Can you work these out from the model? Positions are in its coordinate system, mm. Face numbers are marked on the shaded views. A direction names the side the tool comes from. Give positions to 0.01 mm unless a question says otherwise; leave off trailing zeros. Order: outer loops, then holes, each group sorted by start corner. A loop starts at its lowest first (then second) coordinate and runs counter-clockwise, first axis right, second up. Notation, with made-up numbers: (23, 53) - (69, 53) arc R27 cw to (69, 75) - close; hole circle Ø3 at (81, -6.75). An arc over 180 degrees is marked (long way). Write each question's results on one line, items separated by ' | '. Start each with the question number.
from build123d import *

# Parameters (mm, degrees)
SKETCH1_W                    = 838.2
SKETCH1_H                    = 101.6
BASE_FLANGE1_DEPTH           = 3.175
EDGE_FLANGE1_STRIP_W         = 19.05
EDGE_FLANGE1_STRIP_H         = 3.175
EDGE_FLANGE1_STRIP_CUT_DEPTH = 838.2
EDGE_FLANGE1_DEPTH           = 838.2


# Sheet-metal steps are written as plain solids
with BuildPart() as part:
    # Sketch1 → Base-Flange1 (new body)
    with BuildSketch(Plane(origin=(0, 0, 0), x_dir=(1, 0, 0), z_dir=(0, 1, 0))):
        with Locations((419.1, 50.8)):
            Rectangle(SKETCH1_W, SKETCH1_H)
    extrude(amount=-BASE_FLANGE1_DEPTH)

    # Edge-Flange1 strip (across the edge) → Edge-Flange1 strip cut (cut)
    with BuildSketch(Plane(origin=(0, 0, 0), x_dir=(0, 0, -1), z_dir=(1, 0, 0))):
        with Locations((-3.175, -1.5875)):
            Rectangle(EDGE_FLANGE1_STRIP_W, EDGE_FLANGE1_STRIP_H)
    extrude(amount=EDGE_FLANGE1_STRIP_CUT_DEPTH, mode=Mode.SUBTRACT)

    # Edge-Flange1 section (across the edge) → Edge-Flange1 (add)
    with BuildSketch(Plane(origin=(0, 0, 0), x_dir=(0, 0, -1), z_dir=(1, 0, 0))):
        with BuildLine():
            Line((0, 3.175), (0, 38.1))
            Line((0, 38.1), (3.175, 38.1))
            Line((3.175, 38.1), (3.175, 3.175))
            ThreePointArc((3.175, 3.175), (4.10493597, 0.92993597), (6.35, 0))
            Line((6.35, 0), (6.35, -3.175))
            ThreePointArc((6.35, -3.175), (1.859871939, -1.315128061), (0, 3.175))
        make_face()
    extrude(amount=EDGE_FLANGE1_DEPTH)


solid = part.part
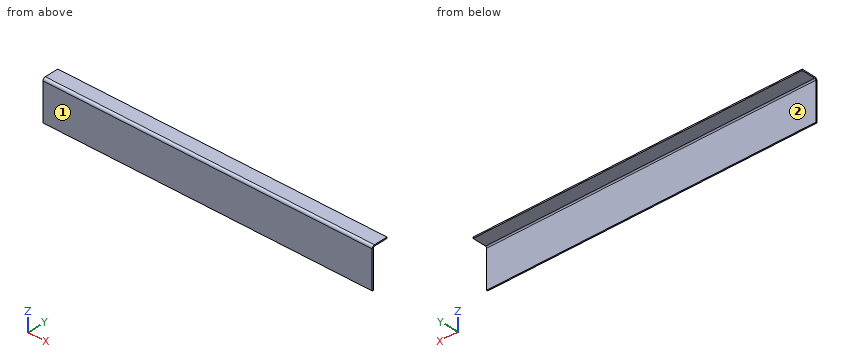
Q1. Will these pins go through, and if not, where does the flat tip stop? P1, Ø4, axis at x = 105.5, y = 3, coming from the -Z side; P2, Ø12, axis at x = 668, y = 15.5, coming from the -Z side (3 decimals); P3, Ø10, axis at x = 630, z = -37.5, coming from the +Y side; P4, Ø1, axis at x = 515.5, y = 16, coming from the +Z side.
Q2. If I drill on probe 1 along Y at (x, z) = (665, -60) (3 decimals); probe 2 along Y at (x, z) = (498, -5.5), over which ranges is the centre line in solid material (lowest first)? Write a range as from..to.
Q3. Which directions (+Z, -Z, +X, -X, +Y, -Y) give clear straight access to the entire face, cutting with the end or side of a thin tool? Please do the marked faces 1 and 2.
Q4. If we section it at B-B (y = 25): Please give me the cut outline in (x, z) (3 decimals).
Q5. If we section it at A-A (x = 302.5): Please give me the cut outline in (y, z) (3 decimals).
Findings below:
1) P1: stops at z = -4.04 | P2: stops at z = -3.175 | P3: stops at y = 0 | P4: stops at z = 0
2) probe 1: y = -3.175..0 | probe 2: y = -3.12..0.12
3) face 1: +Z, -Z, +X, -X, -Y | face 2: -Z, +X, -X, +Y
4) outline: (0, -3.175) - (838.2, -3.175) - (838.2, 0) - (0, 0) - close
5) outline: (-3.175, -101.6) - (0, -101.6) - (0, -6.35) arc R3.175 cw to (3.175, -3.175) - (38.1, -3.175) - (38.1, 0) - (3.175, 0) arc R6.35 ccw to (-3.175, -6.35) - close
